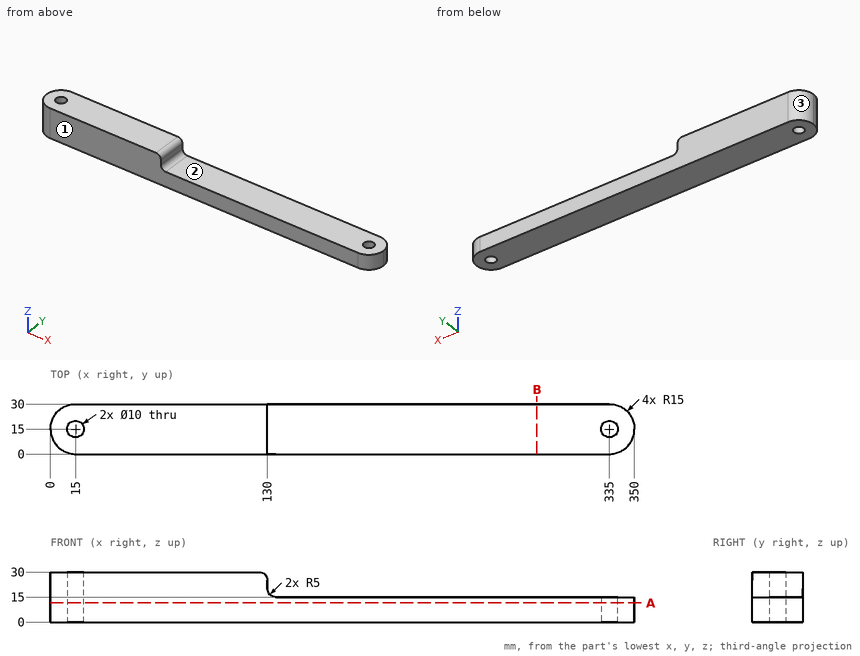
Study the drawing (mm; zero at the part's minimum x, y, z) and answer. Round coordinates to 2 decimals unless told otherwise and drop trailing zeros. Loops run counter-clockwise (first coordinate to the right, second up) from the corner with the lowest first, then second, coordinate; pieces in that order, holes last.
Q1. Given pin 1 Ø1.5 at (y, z) = (19.5, 21.5) entering from +X; pin 2 Ø6 at (x, y) = (15, 15) entering from -Z; pin 3 Ø4 at (x, y) = (311, 24) entering from +Z, each flat-ended and moving along its own axis, determine where each tip first touches the part or whether it passes through.
Q2. Section B-B, the plane x = 291.5 is taken. Determine the outline of the cut face in (y, z), then the cut area to 3 significant figures.
Q3. For a pull along Y with two mould halves and no side action, classify the marked faces 1, 2 and 3 as released by +Y, released by -Y, zero draft, split by the parting line, or undercut.
Q4. Section A-A, the plane z = 11.5 is taken. Count the separate pieces of the cut face and the enclosed holes in it, then the cut area to 3 significant figures.
Q5. Find the intervals of material crossed by line 1 (Y direction, x = 335, z = 10.25); line 2 (X direction, y = 14.5, z = 21.25) (1 decimal); line 3 (X direction, y = 16.5, z = 14.75) (1 decimal), in increasing order.
Completed:
1. pin 1: stops at x = 130
1. pin 2: passes through
1. pin 3: stops at z = 15
2. outline: (0, 0) - (30, 0) - (30, 15) - (0, 15) - close
2. area: 450 mm2
3. face 1: released by -Y
3. face 2: zero draft
3. face 3: released by +Y
4. separate pieces: 1
4. enclosed holes: 2
4. area: 10,100 mm2
5. line 1: y = 0 to 10, 20 to 30
5. line 2: x = 0 to 10, 20 to 130
5. line 3: x = 0.1 to 10.2, 19.8 to 330.2, 339.8 to 349.9
